Here's how the part is built. I have some questions about the finished solid (model axes, mm). A direction names the side the tool comes from. Coordinates: 2 decimals unless noted, no trailing zeros. Use a Markdown table: item, result. Add a question column.
Item 1: If we mould it in two halves opening along X, with no side actions, what happens to faces 4 (the flat face through (23, 68, 0)), 5 (the flat face through (40, 135, -21.81)), 6 (the flat face through (0, 68, -12))? For each: pulls with the +X half, pulls with the -X half, needs draft (parallel to the pull), parting line crosses it, or undercut.
Item 2: On a 3-axis mill with a long thin cutter (end or side, diameter ignored), from which of +Z, -Z, +X, -X, +Y, -Y can I reach the whole of each face in a straight line? I mean faces 1 (the flat face through (3, 135, -23)), 2 (the flat face through (23, 0, -13)), 3 (the cylindrical face through (41.381, 134.549, -24.355)). Say none if no direction works.
Item 3: Will this pin go through, and if not, where does the flat tip stop? pin 1 Ø2 at (x, y) = (6, 133) entering from -Z.
```python
from build123d import *

# Parameters (mm, degrees)
SKETCH1_W           = 47
SKETCH1_H           = 25
BOSS_EXTRUDE1_DEPTH = 138
SKETCH2_W           = 9.48
SKETCH2_H           = 4.865
SKETCH2_R           = 2.0575
SKETCH2_W_2         = 8.82
SKETCH2_H_2         = 3.19
SKETCH2_R_2         = 1.22
CUT_EXTRUDE1_DEPTH  = 7


with BuildPart() as part:
    # Sketch1 → Boss-Extrude1 (new body)
    with BuildSketch(Plane(origin=(0, 0, 0), x_dir=(1, 0, 0), z_dir=(0, 1, 0))):
        with Locations((23.5, 12.5)):
            Rectangle(SKETCH1_W, SKETCH1_H)
    extrude(amount=BOSS_EXTRUDE1_DEPTH)

    # Sketch2 → Cut-Extrude1 (cut)
    with BuildSketch(Plane(origin=(0, 138, 0), x_dir=(1, 0, 0), z_dir=(0, 1, 0))):
        with Locations((7.74, 22.5675)):
            Rectangle(SKETCH2_W, SKETCH2_H)
        with Locations((5.5575, 22.6925)):
            Circle(SKETCH2_R, mode=Mode.SUBTRACT)
        with Locations((9.9225, 22.6925)):
            Circle(SKETCH2_R, mode=Mode.SUBTRACT)
        with Locations((39.59, 23.405)):
            Rectangle(SKETCH2_W_2, SKETCH2_H_2)
        with Locations((36.9, 23.53)):
            Circle(SKETCH2_R_2, mode=Mode.SUBTRACT)
        with Locations((39.59, 23.53)):
            Circle(SKETCH2_R_2, mode=Mode.SUBTRACT)
        with Locations((42.28, 23.53)):
            Circle(SKETCH2_R_2, mode=Mode.SUBTRACT)
    extrude(amount=-CUT_EXTRUDE1_DEPTH, mode=Mode.SUBTRACT)


solid = part.part
```
Ans:
| question | item | result |
|---|---|---|
| 1 | face 4 | needs draft |
| 1 | face 5 | undercut |
| 1 | face 6 | pulls with the -X half |
| 2 | face 1 | -Z, +Y |
| 2 | face 2 | +Z, -Z, +X, -X, -Y |
| 2 | face 3 | +Y |
| 3 | pin 1 | stops at z = -24.75 |
